Source: three-view drawing plus pictorial views. Frame: mm from the lowest corner of the part. A direction names the side the tool comes from. Give positions to 0.01 mm unless a question says otherwise; leave off trailing zeros. Loops run counter-clockwise (first coordinate to the right, second up) from the corner with the lowest first, then second, coordinate; pieces in that order, holes last. Notation, with made-up numbers: (67.25, 86) -> (78.25, 86) arc R23 cw to (78.25, 125) -> close; hole circle Ø4 at (86, -22.75). An arc over 180 degrees is marked (long way). Answer in a Markdown table with one row per item. Add a question column.
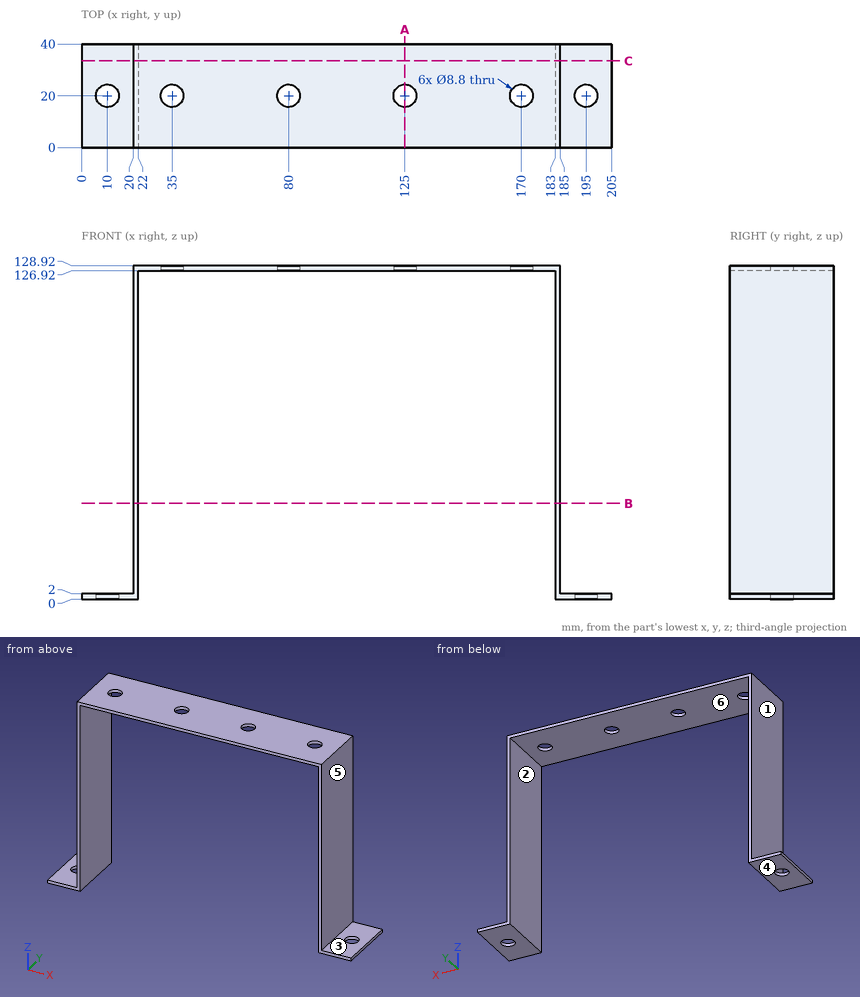
(1) Cut plane B-B on z = 37. Return the cut outline in (x, y), then the cut area to 3 significant figures.
(2) Cut plane A-A on x = 125. Return the cut outline in (y, z).
(3) Material intervals for line 1 along Y through (x, z) = (10, 1.4); line 2 along X through (y, z) = (23, 76.5); line 3 along Z through (x, y) = (42, 6), sorted ascending. Write a range as from..to.
(4) Pin query (flat end, axial travel): pin 1 Ø4 at (y, z) = (33.5, 115.5) entering from +X; pin 2 Ø10 at (x, y) = (158.5, 10.5) entering from -Z; pin 3 Ø10 at (y, z) = (33.5, 16) entering from -X; pin 4 Ø10 at (x, y) = (10, 20) entering from -Z. Return the tip coordinate at first contact, or that it passes through.
(5) Cut plane C-C on y = 33.5. Return the cut outline in (x, z).
(6) Reachability of the marked faces 1, 2 and 3 from +Z, -Z, +X, -X, +Y, -Y: full face, straight path, thin tool, end or side. Return the list, or none.
(7) Draft query along X for the marked faces 4, 5 and 6. Return one class per face: +X half, -X half, draft (parallel to the pull), parting line (faces both ways), or undercut.
Answer list:
| question | item | result |
|---|---|---|
| 1 | outline | (20, 0) -> (22, 0) -> (22, 40) -> (20, 40) -> close; (183, 0) -> (185, 0) -> (185, 40) -> (183, 40) -> close |
| 1 | area | 160 mm² |
| 2 | outline | (0, 126.92) -> (15.6, 126.92) -> (15.6, 128.92) -> (0, 128.92) -> close; (24.4, 126.92) -> (40, 126.92) -> (40, 128.92) -> (24.4, 128.92) -> close |
| 3 | line 1 | y = 0..15.6, 24.4..40 |
| 3 | line 2 | x = 20..22, 183..185 |
| 3 | line 3 | z = 126.92..128.92 |
| 4 | pin 1 | stops at x = 185 |
| 4 | pin 2 | stops at z = 126.92 |
| 4 | pin 3 | stops at x = 20 |
| 4 | pin 4 | stops at z = 0 |
| 5 | outline | (0, 0) -> (22, 0) -> (22, 126.92) -> (183, 126.92) -> (183, 0) -> (205, 0) -> (205, 2) -> (185, 2) -> (185, 128.92) -> (20, 128.92) -> (20, 2) -> (0, 2) -> close |
| 6 | face 1 | +Z, -X, +Y, -Y |
| 6 | face 2 | -Z, +Y, -Y |
| 6 | face 3 | +Z, +X, +Y, -Y |
| 7 | face 4 | draft |
| 7 | face 5 | +X half |
| 7 | face 6 | undercut |
